The listing builds one solid part. Answer for the finished solid, in the listing's coordinates (mm). Round coordinates to 2 decimals unless told otherwise and drop trailing zeros. Order: outer loops, then holes, each group sorted by start corner. A loop starts at its lowest first (then second) coordinate and runs counter-clockwise, first axis right, second up. Notation, with made-up numbers: (-13, 20) -> (5, 20) arc R4 ccw to (5, 26) -> close; hole circle Ø1 at (5, 81). An arc over 180 degrees is marked (long way). Answer in a Markdown table with one row per item. Add a question column.
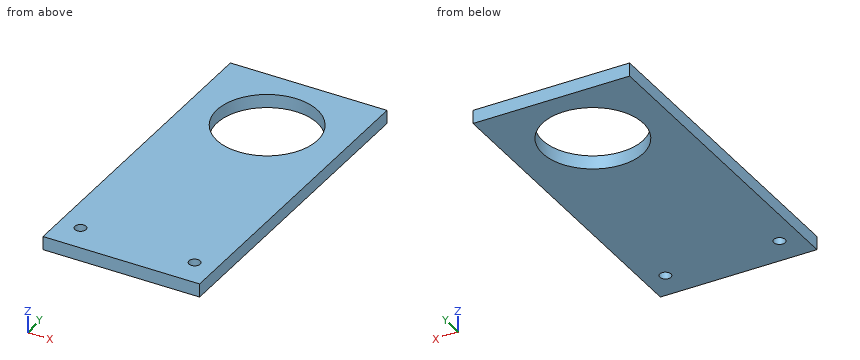
```python
from build123d import *

# Parameters (mm, degrees)
SKETCH2_R           = 22.5
BOSS_EXTRUDE1_DEPTH = 3
SKETCH3_R           = 2.5
CUT_EXTRUDE1_DEPTH  = 6


with BuildPart() as part:
    # Sketch2 → Boss-Extrude1 (new, symmetric)
    with BuildSketch(Plane.XY):
        Polygon((-35, 0), (35, 0), (35, 114), (35, 146.5), (-35, 146.5), (-35, 114), align=None)
        with Locations((0, 114)):
            Circle(SKETCH2_R, mode=Mode.SUBTRACT)
    extrude(amount=BOSS_EXTRUDE1_DEPTH, both=True)

    # Sketch3 → Cut-Extrude1 (cut)
    with BuildSketch(Plane.XY.offset(3)):
        with Locations((-25.5, 12.7)):
            Circle(SKETCH3_R)
        with Locations((25.5, 12.7)):
            Circle(SKETCH3_R)
    extrude(amount=-CUT_EXTRUDE1_DEPTH, mode=Mode.SUBTRACT)


solid = part.part
```
1. The part is cut by section C-C (y = 114). Give the vertices of the cut face in (x, z), then the cut area to 3 significant figures.
2. This flat-tipped pin is pushed along its axis until it touches: pin 1 (4 mm diameter, centred on x = 25.5, y = 12.7, fed in from +Z). Where does it stop, or does it pass through?
3. The part is cut by section A-A (z = -0.5). Give the vertices of the cut face in (x, y), then the cut area to 3 significant figures.
4. Straight lines are drawn through the part: line 1 along Y through (x, z) = (25.5, 0.3); line 2 along Y through (x, z) = (0, -1.55); line 3 along X through (y, z) = (98, -1.75). For each, find the intervals that lie inside material, in ascending order.
5. The part is cut by section D-D (y = 12.7). Give the vertices of the cut face in (x, z).
6. The part is cut by section B-B (x = -25.5). Give the vertices of the cut face in (y, z).
Report:
| question | item | result |
|---|---|---|
| 1 | outline | (-35, -3) -> (-22.5, -3) -> (-22.5, 3) -> (-35, 3) -> close; (22.5, -3) -> (35, -3) -> (35, 3) -> (22.5, 3) -> close |
| 1 | area | 150 mm^2 |
| 2 | pin 1 | passes through |
| 3 | outline | (-35, 0) -> (35, 0) -> (35, 146.5) -> (-35, 146.5) -> close; hole circle Ø5 at (-25.5, 12.7); hole circle Ø45 at (0, 114); hole circle Ø5 at (25.5, 12.7) |
| 3 | area | 8,630 mm^2 |
| 4 | line 1 | y = 0 to 10.2, 15.2 to 146.5 |
| 4 | line 2 | y = 0 to 91.5, 136.5 to 146.5 |
| 4 | line 3 | x = -35 to -15.82, 15.82 to 35 |
| 5 | outline | (-35, -3) -> (-28, -3) -> (-28, 3) -> (-35, 3) -> close; (-23, -3) -> (23, -3) -> (23, 3) -> (-23, 3) -> close; (28, -3) -> (35, -3) -> (35, 3) -> (28, 3) -> close |
| 6 | outline | (0, -3) -> (10.2, -3) -> (10.2, 3) -> (0, 3) -> close; (15.2, -3) -> (146.5, -3) -> (146.5, 3) -> (15.2, 3) -> close |
